The drawing under review shows one solid part. Ordinate dimensions are in mm from its lowest x, y, z. A direction names the side the tool comes from. Coordinates: 2 decimals unless noted, no trailing zeros. Order: outer loops, then holes, each group sorted by start corner. A loop starts at its lowest first (then second) coordinate and runs counter-clockwise, first axis right, second up.
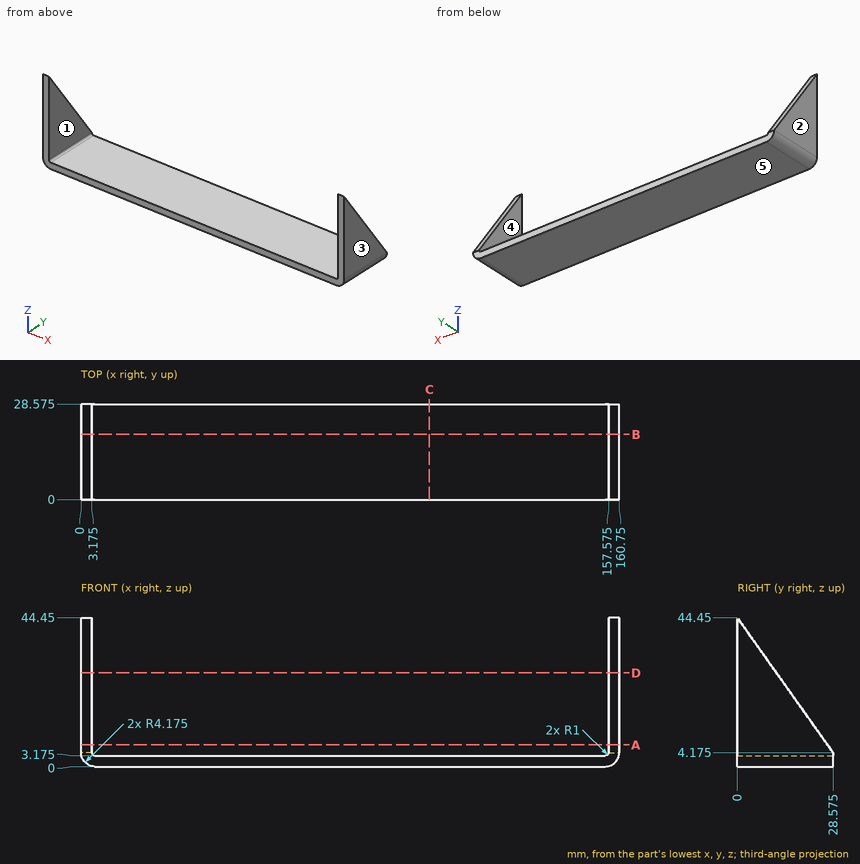
1. Machinability: for the marked faces 1 and 2, which of the approach directions +Z, -Z, +X, -X, +Y, -Y give a long, thin tool a straight path to every point of the face, cutting with its end or side? Answer none if there is none.
Answer below:
face 1: +Z, +Y, -Y
face 2: +Z, -Z, -X, +Y, -Y
2. Take a section at D-D, the plane z = 28. Give the boundary of the cut face in (x, y) (3 decimals).
Answer below:
outline: (0, 0) - (3.175, 0) - (3.175, 11.671) - (0, 11.671) - close; (157.575, 0) - (160.75, 0) - (160.75, 11.671) - (157.575, 11.671) - close
3. Take a section at A-A, the plane z = 6.5. Give the boundary of the cut face in (x, y) (3 decimals), plus the area to 3 significant figures.
Answer below:
outline: (0, 0) - (3.175, 0) - (3.175, 26.925) - (0, 26.925) - close; (157.575, 0) - (160.75, 0) - (160.75, 26.925) - (157.575, 26.925) - close
area: 171 mm2
4. To check wall thickness, follow L1, parallel to X at y = 12.5, z = 26 (3 decimals); L2, parallel to X at y = 3.5, z = 4; L3, parallel to Z at x = 34, y = 21.25 (3 decimals). State the ranges of each line that lie inside material, in increasing order.
Answer below:
L1: x = 0 to 3.175, 157.575 to 160.75
L2: x = 0 to 3.19, 157.56 to 160.75
L3: z = 0 to 3.175
5. Take a section at B-B, the plane y = 19.5. Give the boundary of the cut face in (x, z) (3 decimals).
Answer below:
outline: (0, 4.175) arc R4.175 ccw to (4.175, 0) - (156.575, 0) arc R4.175 ccw to (160.75, 4.175) - (160.75, 16.966) - (157.575, 16.966) - (157.575, 4.175) arc R1 cw to (156.575, 3.175) - (4.175, 3.175) arc R1 cw to (3.175, 4.175) - (3.175, 16.966) - (0, 16.966) - close
6. The part is to be moulded in two halves that separate along X. For the marked faces 3, 4 and 5, say which applies: +X half, -X half, draft (parallel to the pull), parting line (faces both ways), or undercut.
Answer below:
face 3: +X half
face 4: undercut
face 5: draft
7. Clearance check with a flat-ended pin moving along its axis: pin 1 Ø2 at (x, y) = (73.5, 13) entering from +Z (3 decimals). State where the tip first meets the part, or that it passes through.
Answer below:
pin 1: stops at z = 3.175
8. Take a section at C-C, the plane x = 104. Give the boundary of the cut face in (y, z) (3 decimals).
Answer below:
outline: (0, 0) - (28.575, 0) - (28.575, 3.175) - (0, 3.175) - close
